Work out the finished part from the listing and answer in its coordinate system (mm). Face numbers are marked on the shaded views. A direction names the side the tool comes from. Coordinates: 2 decimals unless noted, no trailing zeros. Loops run counter-clockwise (first coordinate to the right, second up) from the corner with the lowest first, then second, coordinate; pieces in that order, holes last. Notation, with made-up numbers: (-8.75, 39) -> (19.25, 39) arc R29 ccw to (19.25, 73) -> close; hole circle Ø4 at (18.25, 42). An arc over 180 degrees is marked (long way). Use a Markdown table: item, result.
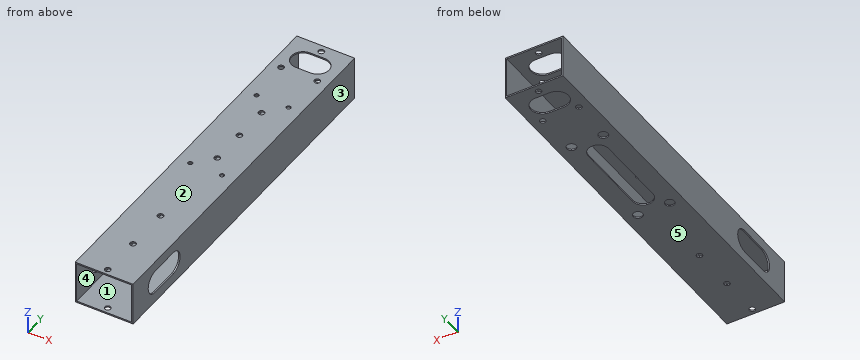
from build123d import *

# Parameters (mm, degrees)
SKETCH_1_W               = 40
SKETCH_1_H               = 30
EXTRUDE_1_DEPTH          = 125
SKETCH_2_W               = 38
SKETCH_2_H               = 28
CUT_EXTRUDE_1_DEPTH      = 126
CUT_EXTRUDE_1_DEPTH_BACK = 126
SKETCH_3_R               = 2.025
CUT_EXTRUDE_2_DEPTH      = 1
CUT_EXTRUDE_2_DEPTH_BACK = 31
SKETCH_4_R               = 2.025
CUT_EXTRUDE_3_DEPTH      = 1
CUT_EXTRUDE_3_DEPTH_BACK = 31
SKETCH_5_R               = 1.525
CUT_EXTRUDE_4_DEPTH      = 31
SKETCH_6_R               = 2.025
CUT_EXTRUDE_5_DEPTH      = 31
CUT_EXTRUDE_6_DEPTH      = 10
SKETCH_8_R               = 3.25
CUT_EXTRUDE_7_DEPTH      = 10
CUT_EXTRUDE_8_DEPTH      = 1
CUT_EXTRUDE_8_DEPTH_BACK = 41
CUT_EXTRUDE_9_DEPTH      = 1
CUT_EXTRUDE_9_DEPTH_BACK = 31


with BuildPart() as part:
    # 草图1 → 凸台-拉伸1 (new body, symmetric)
    with BuildSketch(Plane(origin=(0, 0, 0), x_dir=(1, 0, 0), z_dir=(0, 1, 0))):
        Rectangle(SKETCH_1_W, SKETCH_1_H)
    extrude(amount=EXTRUDE_1_DEPTH, both=True)

    # 草图2 → 切除-拉伸1 (cut, two sides)
    with BuildSketch(Plane(origin=(0, 0, 0), x_dir=(1, 0, 0), z_dir=(0, 1, 0))) as cut_extrude_1_sk:
        Rectangle(SKETCH_2_W, SKETCH_2_H)
    extrude(amount=CUT_EXTRUDE_1_DEPTH, mode=Mode.SUBTRACT)
    extrude(cut_extrude_1_sk.sketch, amount=-CUT_EXTRUDE_1_DEPTH_BACK, mode=Mode.SUBTRACT)

    # 草图3 → 切除-拉伸2 (cut, two sides)
    with BuildSketch(Plane.XY.offset(15)) as cut_extrude_2_sk:
        with Locations((0, -61.5)):
            Circle(SKETCH_3_R)
        with Locations((0, -92.5)):
            Circle(SKETCH_3_R)
        with Locations((0, -121)):
            Circle(SKETCH_3_R)
    extrude(amount=CUT_EXTRUDE_2_DEPTH, mode=Mode.SUBTRACT)
    extrude(cut_extrude_2_sk.sketch, amount=-CUT_EXTRUDE_2_DEPTH_BACK, mode=Mode.SUBTRACT)

    # 草图4 → 切除-拉伸3 (cut, two sides)
    with BuildSketch(Plane(origin=(0, 0, -15), x_dir=(-1, 0, 0), z_dir=(0, 0, -1))) as cut_extrude_3_sk:
        with Locations((0, 120)):
            Circle(SKETCH_4_R)
        with Locations((-12.5, 95)):
            Circle(SKETCH_4_R)
        with Locations((12.5, 95)):
            Circle(SKETCH_4_R)
    extrude(amount=CUT_EXTRUDE_3_DEPTH, mode=Mode.SUBTRACT)
    extrude(cut_extrude_3_sk.sketch, amount=-CUT_EXTRUDE_3_DEPTH_BACK, mode=Mode.SUBTRACT)

    # 草图5 → 切除-拉伸4 (cut, through all)
    with BuildSketch(Plane(origin=(0, 0, -15), x_dir=(-1, 0, 0), z_dir=(0, 0, -1))):
        with Locations((-11, 65)):
            Circle(SKETCH_5_R)
        with Locations((11, 65)):
            Circle(SKETCH_5_R)
        with Locations((-11, -10)):
            Circle(SKETCH_5_R)
        with Locations((11, -10)):
            Circle(SKETCH_5_R)
    extrude(amount=-CUT_EXTRUDE_4_DEPTH, mode=Mode.SUBTRACT)

    # 草图6 → 切除-拉伸5 (cut, through all)
    with BuildSketch(Plane(origin=(0, 0, -15), x_dir=(-1, 0, 0), z_dir=(0, 0, -1))):
        with Locations((0, 27.5)):
            Circle(SKETCH_6_R)
        with Locations((0, 52.5)):
            Circle(SKETCH_6_R)
        with Locations((0, 2.5)):
            Circle(SKETCH_6_R)
    extrude(amount=-CUT_EXTRUDE_5_DEPTH, mode=Mode.SUBTRACT)

    # 草图7 → 切除-拉伸6 (cut)
    with BuildSketch(Plane(origin=(0, 0, -15), x_dir=(-1, 0, 0), z_dir=(0, 0, -1))):
        with BuildLine():
            Line((7, 52.5), (7, 2.5))
            ThreePointArc((7, 2.5), (0, -4.5), (-7, 2.5))
            Line((-7, 2.5), (-7, 52.5))
            ThreePointArc((-7, 52.5), (0, 59.5), (7, 52.5))
        make_face()
    extrude(amount=-CUT_EXTRUDE_6_DEPTH, mode=Mode.SUBTRACT)

    # 草图8 → 切除-拉伸7 (cut)
    with BuildSketch(Plane(origin=(0, 0, -15), x_dir=(-1, 0, 0), z_dir=(0, 0, -1))):
        with Locations((11, 65)):
            Circle(SKETCH_8_R)
        with Locations((-11, 65)):
            Circle(SKETCH_8_R)
        with Locations((11, -10)):
            Circle(SKETCH_8_R)
        with Locations((-11, -10)):
            Circle(SKETCH_8_R)
    extrude(amount=-CUT_EXTRUDE_7_DEPTH, mode=Mode.SUBTRACT)

    # 草图9 → 切除-拉伸8 (cut, two sides)
    with BuildSketch(Plane(origin=(20, 0, 0), x_dir=(0, 0, -1), z_dir=(1, 0, 0))) as cut_extrude_8_sk:
        with BuildLine():
            Line((-8, -100), (-8, -80))
            ThreePointArc((-8, -80), (0, -72), (8, -80))
            Line((8, -80), (8, -100))
            ThreePointArc((8, -100), (0, -108), (-8, -100))
        make_face()
    extrude(amount=CUT_EXTRUDE_8_DEPTH, mode=Mode.SUBTRACT)
    extrude(cut_extrude_8_sk.sketch, amount=-CUT_EXTRUDE_8_DEPTH_BACK, mode=Mode.SUBTRACT)

    # 草图10 → 切除-拉伸9 (cut, two sides)
    with BuildSketch(Plane(origin=(0, 0, -15), x_dir=(-1, 0, 0), z_dir=(0, 0, -1))) as cut_extrude_9_sk:
        with BuildLine():
            Line((-5, 115.5), (5, 115.5))
            ThreePointArc((5, 115.5), (13, 107.5), (5, 99.5))
            Line((5, 99.5), (-5, 99.5))
            ThreePointArc((-5, 99.5), (-13, 107.5), (-5, 115.5))
        make_face()
    extrude(amount=CUT_EXTRUDE_9_DEPTH, mode=Mode.SUBTRACT)
    extrude(cut_extrude_9_sk.sketch, amount=-CUT_EXTRUDE_9_DEPTH_BACK, mode=Mode.SUBTRACT)


solid = part.part
Q1. Determine the mould class of the marked faces 3, 4 and 5 for opening direction X: pulls with the +X half, pulls with the -X half, needs draft (parallel to the pull), parting line crosses it, or undercut.
Solved:
| item | result |
|---|---|
| face 3 | pulls with the +X half |
| face 4 | undercut |
| face 5 | needs draft |
Q2. For the marked faces 1 and 2, determine the directions among +Z, -Z, +X, -X, +Y, -Y from which every point of the face is accessible in a straight line to the end or side of a thin tool.
Solved:
| item | result |
|---|---|
| face 1 | +Y, -Y |
| face 2 | +Z, +X, -X, +Y, -Y |
Q3. Section A-A on y = 107.5 is taken. Determine the outline of the cut face in (x, z).
Solved:
| item | result |
|---|---|
| outline | (-20, -15) -> (-13, -15) -> (-13, -14) -> (-19, -14) -> (-19, 14) -> (-13, 14) -> (-13, 15) -> (-20, 15) -> close; (13, -15) -> (20, -15) -> (20, 15) -> (13, 15) -> (13, 14) -> (19, 14) -> (19, -14) -> (13, -14) -> close |
Q4. Section C-C on y = -49.5 is taken. Determine the outline of the cut face in (x, z), and give its area (3 significant figures).
Solved:
| item | result |
|---|---|
| outline | (-20, -15) -> (20, -15) -> (20, 15) -> (-20, 15) -> close; hole (-19, -14) -> (19, -14) -> (19, 14) -> (-19, 14) -> close |
| area | 136 mm² |
Q5. Given pin 1 Ø10 at (x, z) = (-10, -8.5) entering from +Y, flat-ended and moving along its own axis, determine where the tip first touches the part or whether it passes through.
Solved:
| item | result |
|---|---|
| pin 1 | through |
Q6. Section B-B on z = 11.5 is taken. Determine the outline of the cut face in (x, y).
Solved:
| item | result |
|---|---|
| outline | (-20, -125) -> (-19, -125) -> (-19, 125) -> (-20, 125) -> close; (19, -125) -> (20, -125) -> (20, 125) -> (19, 125) -> close |
Q7. Consider line 1 (Z direction, x = 2.5, y = -29); line 2 (X direction, y = 65, z = 14.65) (3 decimals); line 3 (X direction, y = 27, z = 0.5). Determine where each line is inside the solid, lowest interval first. Write a range as [from, to].
Solved:
| item | result |
|---|---|
| line 1 | [-15, -14], [14, 15] |
| line 2 | [-20, -12.525], [-9.475, 9.475], [12.525, 20] |
| line 3 | [-20, -19], [19, 20] |
Q8. Section D-D on z = -4 is taken. Determine the outline of the cut face in (x, y), and give its area (3 significant figures).
Solved:
| item | result |
|---|---|
| outline | (-20, -125) -> (-19, -125) -> (-19, -106.93) -> (-20, -106.93) -> close; (-20, -73.07) -> (-19, -73.07) -> (-19, 125) -> (-20, 125) -> close; (19, -125) -> (20, -125) -> (20, -106.93) -> (19, -106.93) -> close; (19, -73.07) -> (20, -73.07) -> (20, 125) -> (19, 125) -> close |
| area | 432 mm² |
